from build123d import *

# Parameters (mm, degrees)
SKETCH1_W           = 90
SKETCH1_H           = 40
BOSS_EXTRUDE1_DEPTH = 5
BOSS_EXTRUDE2_DEPTH = 12
SKETCH3_W           = 5
SKETCH3_H           = 40
BOSS_EXTRUDE3_DEPTH = 10
SKETCH5_R           = 2.125
CUT_EXTRUDE1_DEPTH  = 91
SKETCH7_R           = 1.25
CUT_EXTRUDE3_DEPTH  = 35
SKETCH8_W           = 10
SKETCH8_H           = 0.75
CUT_EXTRUDE4_DEPTH  = 91
SKETCH12_R          = 1.5
CUT_EXTRUDE6_DEPTH  = 28
SKETCH13_R          = 1.25
CUT_EXTRUDE7_DEPTH  = 5


with BuildPart() as part:
    # Sketch1 → Boss-Extrude1 (new body)
    with BuildSketch(Plane(origin=(0, 0, 0), x_dir=(1, 0, 0), z_dir=(0, 1, 0))):
        Rectangle(SKETCH1_W, SKETCH1_H)
    extrude(amount=BOSS_EXTRUDE1_DEPTH)

    # Sketch2 → Boss-Extrude2 (add)
    with BuildSketch(Plane(origin=(0, 5, 0), x_dir=(1, 0, 0), z_dir=(0, 1, 0))):
        Polygon((-21, -20), (-21, -15), (-40, -15), (-40, 15), (-2, 15), (-2, 20), (-45, 20), (-45, -20), align=None)
        Polygon((2, -15), (40, -15), (40, 15), (21, 15), (21, 20), (45, 20), (45, -20), (2, -20), align=None)
    extrude(amount=BOSS_EXTRUDE2_DEPTH)

    # Sketch3 → Boss-Extrude3 (add)
    with BuildSketch(Plane(origin=(0, 17, 0), x_dir=(1, 0, 0), z_dir=(0, 1, 0))):
        with Locations((42.5, 0)):
            Rectangle(SKETCH3_W, SKETCH3_H)
        with Locations((-42.5, 0)):
            Rectangle(SKETCH3_W, SKETCH3_H)
    extrude(amount=BOSS_EXTRUDE3_DEPTH)

    # Sketch5 → Cut-Extrude1 (cut, through all)
    with BuildSketch(Plane.ZY.offset(45)):
        with Locations((16, 23)):
            Circle(SKETCH5_R)
        with Locations((-16, 23)):
            Circle(SKETCH5_R)
    extrude(amount=-CUT_EXTRUDE1_DEPTH, mode=Mode.SUBTRACT)

    # Sketch7 → Cut-Extrude3 (cut)
    with BuildSketch(Plane(origin=(0, 0, 15), x_dir=(-1, 0, 0), z_dir=(0, 0, -1))):
        with Locations((-23.25, 11)):
            Circle(SKETCH7_R)
        with Locations((4.25, 11)):
            Circle(SKETCH7_R)
    extrude(amount=CUT_EXTRUDE3_DEPTH, mode=Mode.SUBTRACT)

    # Sketch8 → Cut-Extrude4 (cut, through all)
    with BuildSketch(Plane.ZY.offset(45)):
        with Locations((15, 23)):
            Rectangle(SKETCH8_W, SKETCH8_H)
        with Locations((-15, 23)):
            Rectangle(SKETCH8_W, SKETCH8_H)
    extrude(amount=-CUT_EXTRUDE4_DEPTH, mode=Mode.SUBTRACT)

    # Sketch12 → Cut-Extrude6 (cut, through all)
    with BuildSketch(Plane.XZ):
        with Locations((-30, 10)):
            Circle(SKETCH12_R)
        with Locations((-30, -10)):
            Circle(SKETCH12_R)
        with Locations((-7, 10)):
            Circle(SKETCH12_R)
        with Locations((-7, -10)):
            Circle(SKETCH12_R)
    extrude(amount=-CUT_EXTRUDE6_DEPTH, mode=Mode.SUBTRACT)

    # Sketch13 → Cut-Extrude7 (cut)
    with BuildSketch(Plane.XY.offset(20)):
        with Locations((-23.25, 11)):
            Circle(SKETCH13_R)
        with Locations((4.25, 11)):
            Circle(SKETCH13_R)
    extrude(amount=-CUT_EXTRUDE7_DEPTH, mode=Mode.SUBTRACT)


solid = part.part
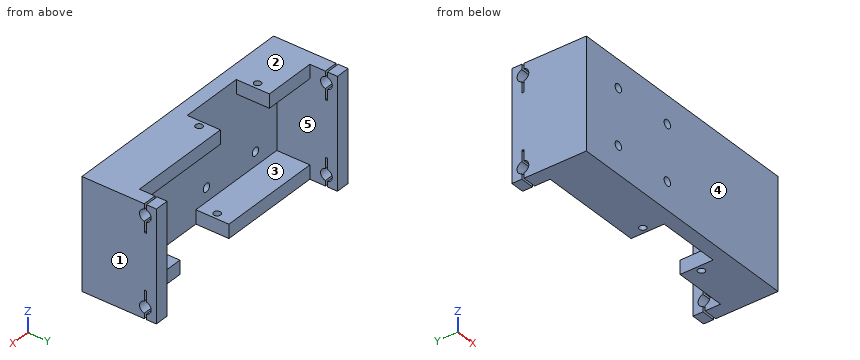
CAD build for the part. Positions are in the model's coordinates, mm. Face numbers are marked on the shaded views. A direction names the side the tool comes from. Coordinates: 2 decimals unless noted, no trailing zeros. Order: outer loops, then holes, each group sorted by start corner. A loop starts at its lowest first (then second) coordinate and runs counter-clockwise, first axis right, second up. Notation, with made-up numbers: (-27, -6) -> (-5, -6) arc R25 cw to (-5, 13) -> close; hole circle Ø5 at (-13, 47). An arc over 180 degrees is marked (long way). Answer in a Markdown table with one row per item.
1) Band-saw the part on A-A (y = 11). Give the number of separate pieces and of enclosed holes in the cut face, and give its area (3 significant figures).
Check values:
| item | result |
|---|---|
| separate pieces | 6 |
| enclosed holes | 0 |
| area | 920 mm2 |
2) Drill centre lines: line 1 (X direction, y = 11, z = -18.9); line 2 (Z direction, x = -30, y = 3.7); line 3 (X direction, y = 11.25, z = 10). Where is each one in solid material? Low to high.
Check values:
| item | result |
|---|---|
| line 1 | -45 to -5.5, -3 to -2, 21 to 22, 24.5 to 45 |
| line 2 | -20 to -11.5, -8.5 to 8.5, 11.5 to 20 |
| line 3 | -45 to -40, 40 to 45 |
3) Band-saw the part on D-D (x = -30). List the corners of the cut face in (y, z).
Check values:
| item | result |
|---|---|
| outline | (0, -20) -> (17, -20) -> (17, -15) -> (5, -15) -> (5, -11.5) -> (0, -11.5) -> close; (0, -8.5) -> (5, -8.5) -> (5, 8.5) -> (0, 8.5) -> close; (0, 11.5) -> (5, 11.5) -> (5, 15) -> (17, 15) -> (17, 20) -> (0, 20) -> close |
4) Which spindle directions (+Z, -Z, +X, -X, +Y, -Y) get a long thin tool onto all of the face, cutting with end or side? Do the marked faces 4 and 5. Say none if no direction does.
Check values:
| item | result |
|---|---|
| face 4 | +Z, -Z, +X, -X, -Y |
| face 5 | +Y |
5) Band-saw the part on B-B (x = 4.25). List the corners of the cut face in (y, z).
Check values:
| item | result |
|---|---|
| outline | (0, -20) -> (5, -20) -> (5, 15) -> (9.75, 15) -> (9.75, 20) -> (0, 20) -> close; (12.25, 15) -> (17, 15) -> (17, 20) -> (12.25, 20) -> close |
6) Band-saw the part on C-C (y = 15.75). List the corners of the cut face in (x, z), and give its area (3 significant figures).
Check values:
| item | result |
|---|---|
| outline | (-45, -20) -> (-2, -20) -> (-2, -15) -> (-40, -15) -> (-40, 15) -> (-21, 15) -> (-21, 20) -> (-45, 20) -> close; (2, 15) -> (40, 15) -> (40, -15) -> (21, -15) -> (21, -20) -> (45, -20) -> (45, 20) -> (2, 20) -> close |
| area | 970 mm2 |
7) Mould opens along X. For the marked faces 1, 2 and 3 say: pulls with the +X half, pulls with the -X half, needs draft (parallel to the pull), parting line crosses it, or undercut.
Check values:
| item | result |
|---|---|
| face 1 | pulls with the +X half |
| face 2 | needs draft |
| face 3 | undercut |
8) Flat gauge pins, fed straight in: P1, Ø5.5, axis at x = 33, z = -16.5, coming from the +Y side; P2, Ø4, axis at x = -7, z = 10, coming from the +Y side. Where does each tip first touch, or does it go through?
Check values:
| item | result |
|---|---|
| P1 | y = 17 |
| P2 | y = 5 |
